Could you check a few things on this drawing? It's one solid part, dimensions in mm from its lowest x, y, z. Give positions to 0.01 mm unless a question says otherwise; leave off trailing zeros. Order: outer loops, then holes, each group sorted by start corner. A loop starts at its lowest first (then second) coordinate and runs counter-clockwise, first axis right, second up.
Item 1: I want a section at B-B, the plane z = 12. Write out the boundary of the cut face in (x, y), then the cut area to 3 significant figures.
Item 2: I want a section at C-C, the plane x = 9. Write out the boundary of the cut face in (y, z).
Item 3: I want a section at A-A, the plane y = 0.4. Write out the boundary of the cut face in (x, z).
Item 4: If I drill on line 1 along X through (y, z) = (1.9, 23), over which ranges is the centre line in solid material (lowest first)?
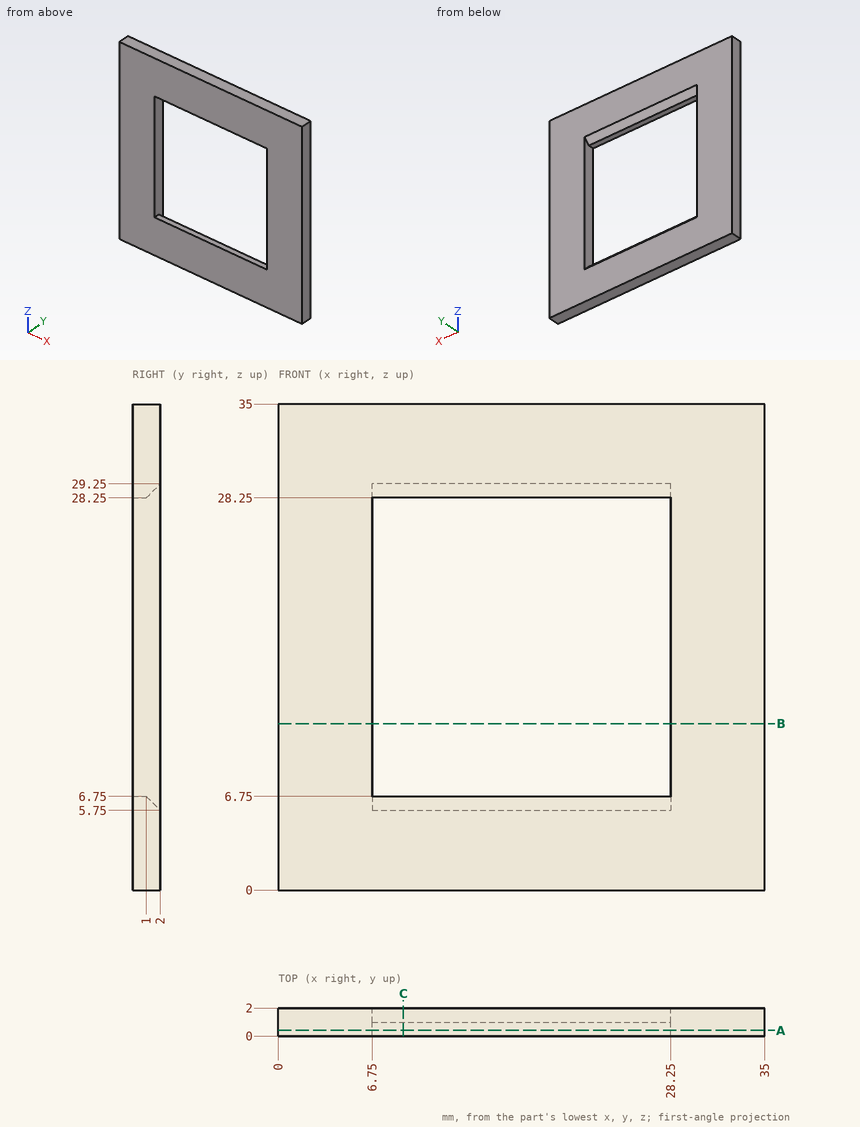
Results list:
1. outline: (0, 0) - (6.75, 0) - (6.75, 2) - (0, 2) - close; (28.25, 0) - (35, 0) - (35, 2) - (28.25, 2) - close
1. area: 27.0 mm2
2. outline: (0, 0) - (2, 0) - (2, 5.75) - (1, 6.75) - (0, 6.75) - close; (0, 28.25) - (1, 28.25) - (2, 29.25) - (2, 35) - (0, 35) - close
3. outline: (0, 0) - (35, 0) - (35, 35) - (0, 35) - close; hole (6.75, 6.75) - (28.25, 6.75) - (28.25, 28.25) - (6.75, 28.25) - close
4. line 1: x = 0 to 6.75, 28.25 to 35
